from build123d import *

# Parameters (mm, degrees)
SKETCH11_W         = 88.1126
SKETCH11_H         = 31.75
SKETCH11_R         = 6.36905
SKETCH11_R_2       = 6.35635
EXTRUDE3_DEPTH     = 11.1125
CUT_EXTRUDE1_DEPTH = 23.7998
FILLET1_R          = 9.525
EXTRUDE4_DEPTH     = 7.9248
SKETCH15_R         = 21.901149079
CUT_EXTRUDE2_DEPTH = 10.525


with BuildPart() as part:
    # Sketch11 → Extrude3 (new body, symmetric)
    with BuildSketch(Plane.XY):
        with Locations((-34.5313, 6.35)):
            Rectangle(SKETCH11_W, SKETCH11_H)
        Circle(SKETCH11_R, mode=Mode.SUBTRACT)
        with Locations((-30.1498, 9.525)):
            Circle(SKETCH11_R_2, mode=Mode.SUBTRACT)
    extrude(amount=EXTRUDE3_DEPTH, both=True)

    # Sketch12 → Cut-Extrude1 (cut)
    with BuildSketch(Plane.XZ.offset(9.525)):
        with BuildLine():
            Line((-12.7127, 5.6769), (9.525, 5.6769))
            Line((9.525, 5.6769), (9.525, -5.6769))
            Line((9.525, -5.6769), (-12.7127, -5.6769))
            ThreePointArc((-12.7127, -5.6769), (-18.3896, 0), (-12.7127, 5.6769))
        make_face()
    extrude(amount=-CUT_EXTRUDE1_DEPTH, mode=Mode.SUBTRACT)

    # Fillet1
    fillet1_edges = [part.edges().sort_by_distance(p)[0] for p in [
        (9.525, -9.525, -8.3947),
        (9.525, -9.525, 8.3947),
    ]]
    fillet(fillet1_edges, radius=FILLET1_R)

    # Sketch13 → Extrude4 (add)
    with BuildSketch(Plane(origin=(0, 22.225, 0), x_dir=(1, 0, 0), z_dir=(0, 1, 0))):
        Polygon((-57.251277372, 0), (-62.750538686, 9.525), (-73.749061314, 9.525), (-79.248322628, 0), (-73.749061314, -9.525), (-62.750538686, -9.525), align=None)
    extrude(amount=EXTRUDE4_DEPTH)

    # Sketch14 → Revolve2 (revolve)
    with BuildSketch(Plane.XY, mode=Mode.PRIVATE) as revolve2_sk:
        with BuildLine():
            Line((-68.2498, 60.200443212), (-73.9648, 63.5))
            Line((-73.9648, 63.5), (-74.5998, 62.865))
            Line((-74.5998, 62.865), (-74.5998, -12.7))
            Line((-74.5998, -12.7), (-90.150949079, -12.7))
            Line((-90.150949079, -12.7), (-90.150949079, -13.462))
            ThreePointArc((-90.150949079, -13.462), (-80.044401519, -19.952955747), (-68.2498, -22.225))
            Line((-68.2498, -22.225), (-68.2498, 60.200443212))
        make_face()
    revolve(revolve2_sk.sketch.rotate(Axis((-68.2498, 26.585218564, 0), (0, -1, 0)), 270), axis=Axis((-68.2498, 26.585218564, 0), (0, -1, 0)))  # turned: the seam where the file's is

    # Sketch15 → Cut-Extrude2 (cut, through all)
    with BuildSketch(Plane(origin=(0, -12.7, 0), x_dir=(1, 0, 0), z_dir=(0, 1, 0))):
        with Locations((-68.2498, 0)):
            Circle(SKETCH15_R)
        Polygon((-68.2498, 8.980256121), (-77.230056121, 0), (-68.2498, -8.980256121), (-59.269543879, 0), align=None, mode=Mode.SUBTRACT)
    extrude(amount=-CUT_EXTRUDE2_DEPTH, mode=Mode.SUBTRACT)


solid = part.part
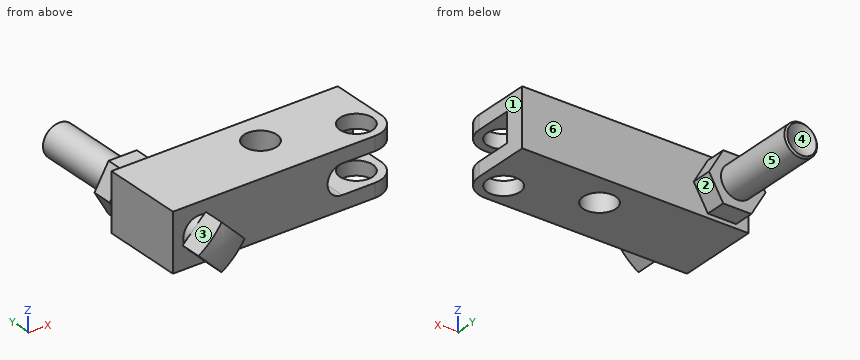
Work out the finished part from the listing and answer in its coordinate system (mm). Face numbers are marked on the shaded views. A direction names the side the tool comes from. Give positions to 0.01 mm unless a question says otherwise; leave off trailing zeros. Loops run counter-clockwise (first coordinate to the right, second up) from the corner with the lowest first, then second, coordinate; pieces in that order, holes last. Notation, with made-up numbers: (30, -34) -> (54, -34) arc R9 ccw to (54, -23) -> close; hole circle Ø11 at (-2.5, 14.25). An arc over 180 degrees is marked (long way). Use a Markdown table: item, result. Add a question column.
1. For the marked faces 1, 2 and 3, determine the directions among +Z, -Z, +X, -X, +Y, -Y from which every point of the face is accessible in a straight line to the end or side of a thin tool.
2. Determine the mould class of the marked faces 4, 5 and 6 for opening direction X: released by +X, released by -X, zero draft, split by the parting line, or undercut.
3. Section A-A on z = -7.75 is taken. Determine the outline of the cut face in (x, y) (3 decimals).
4. Flat-ended cylindrical pins translate along their axes: pin 1 Ø6.5 at (x, y) = (-70, 27) entering from +Z (3 decimals); pin 2 Ø3 at (x, z) = (-53, -3.5) entering from +Y (3 decimals); pin 3 Ø1.5 at (y, z) = (-7.5, 4) entering from -X. Find the tip coordinate at first contact, or state that the pin passes through.
5. Find the intervals of material crossed by probe 1 along X at (y, z) = (0, 8.45) (3 decimals); probe 2 along X at (y, z) = (5, -5.75) (3 decimals); probe 3 along Z at (x, y) = (6.5, -6.5), in increasing order.
6. Section B-B on x = -21 is taken. Determine the outline of the cut face in (y, z) (1 decimal), and give its area (3 significant figures).
Results below:
| question | item | result |
|---|---|---|
| 1 | face 1 | +Z, -Z, +X, +Y, -Y |
| 1 | face 2 | -Z, +X, +Y |
| 1 | face 3 | +Z, -X, -Y |
| 2 | face 4 | undercut |
| 2 | face 5 | split by the parting line |
| 2 | face 6 | zero draft |
| 3 | outline | (-78.588, -9.525) -> (0, -9.525) arc R9.525 ccw to (9.525, 0) -> (9.525, 22.225) -> (-61.726, 22.225) -> (-61.726, 30.15) -> (-74.774, 30.15) -> (-74.774, 22.225) -> (-78.588, 22.225) -> close; (-69.48, -21.24) arc R30.79 ccw to (-67.02, -21.24) -> (-67.02, -12.7) -> (-69.48, -12.7) -> close; hole circle Ø12.713 at (-30.15, 9.525); hole circle Ø12.738 at (0, 0) |
| 4 | pin 1 | stops at z = 9.525 |
| 4 | pin 2 | stops at y = 22.225 |
| 4 | pin 3 | stops at x = -78.59 |
| 5 | probe 1 | x = -78.588 to -6.369, 6.369 to 9.525 |
| 5 | probe 2 | x = -78.588 to -34.614, -25.686 to -3.945, 3.945 to 9.525 |
| 5 | probe 3 | z = -11.11 to -5.68, 5.68 to 11.11 |
| 6 | outline | (-9.5, -11.1) -> (22.2, -11.1) -> (22.2, 11.1) -> (-9.5, 11.1) -> close |
| 6 | area | 706 mm^2 |
